Source: three-view drawing plus pictorial views. Frame: mm from the lowest corner of the part. A direction names the side the tool comes from. Coordinates: 2 decimals unless noted, no trailing zeros. Loops run counter-clockwise (first coordinate to the right, second up) from the corner with the lowest first, then second, coordinate; pieces in that order, holes last. Notation, with made-up numbers: (-12, 57.5) - (42, 57.5) arc R33 cw to (42, 87.5) - close; hole circle Ø8 at (56.5, 10.25). An arc over 180 degrees is marked (long way). Answer as CSV lines item,"result". Start each with the question number.
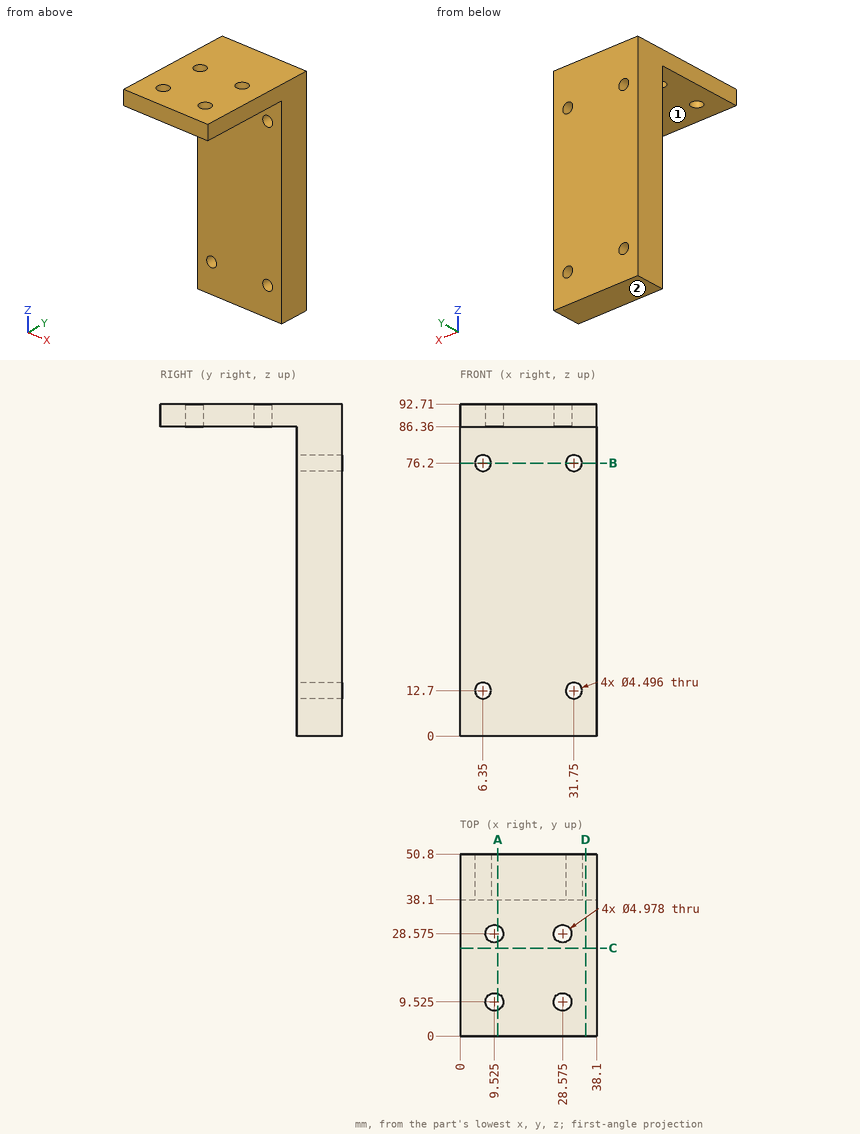
Item 1: Material intervals for probe 1 along X at (y, z) = (44.5, 12.7); probe 2 along X at (y, z) = (44, 12) (1 decimal); probe 3 along Y at (x, z) = (11, 8), sorted ascending.
Item 2: Section query D-D, the plane x = 35. Output: boundary loops of the cut face in (y, z), and give its area (3 significant figures).
Item 3: Set-up query: the marked faces 1 and 2. Return all of +Z, -Z, +X, -X, +Y, -Y with unobstructed straight access to the full face (end or side cutting, diameter ignored); none if empty.
Item 4: Section query C-C, the plane y = 24.5. Output: boundary loops of the cut face in (x, z), and give its area (3 significant figures).
Item 5: Section query A-A, the plane x = 10.5. Output: boundary loops of the cut face in (y, z) (1 decimal).
Item 6: Section query B-B, the plane z = 76.2. Output: boundary loops of the cut face in (x, y), and give its area (3 significant figures).
Item 7: Contact query for flat-ended pins moving along their axis: P1, Ø6, axis at x = 27.5, z = 12, coming from the -Y side; P2, Ø7, axis at x = 6.35, z = 12.7, coming from the +Y side; P3, Ø1, axis at x = 11, y = 11.5, coming from the -Z side. Output: stop coordinate, or through.
Response values:
1,probe 1,"x = 0 to 4.1, 8.6 to 29.5, 34 to 38.1"
1,probe 2,"x = 0 to 4.2, 8.5 to 29.6, 33.9 to 38.1"
1,probe 3,"y = 38.1 to 50.8"
2,outline,"(0, 86.36) - (38.1, 86.36) - (38.1, 0) - (50.8, 0) - (50.8, 92.71) - (0, 92.71) - close"
2,area,"1,420 mm²"
3,face 1,"-Z, +X, -X, -Y"
3,face 2,"-Z, +X, -X, +Y, -Y"
4,outline,"(0, 86.36) - (38.1, 86.36) - (38.1, 92.71) - (0, 92.71) - close"
4,area,"242 mm²"
5,outline,"(0, 86.4) - (7.2, 86.4) - (7.2, 92.7) - (0, 92.7) - close; (11.8, 86.4) - (26.3, 86.4) - (26.3, 92.7) - (11.8, 92.7) - close; (30.9, 86.4) - (38.1, 86.4) - (38.1, 0) - (50.8, 0) - (50.8, 92.7) - (30.9, 92.7) - close"
6,outline,"(0, 38.1) - (4.1, 38.1) - (4.1, 50.8) - (0, 50.8) - close; (8.6, 38.1) - (29.5, 38.1) - (29.5, 50.8) - (8.6, 50.8) - close; (34, 38.1) - (38.1, 38.1) - (38.1, 50.8) - (34, 50.8) - close"
6,area,"370 mm²"
7,P1,"stops at y = 38.1"
7,P2,"stops at y = 50.8"
7,P3,"stops at z = 86.36"
